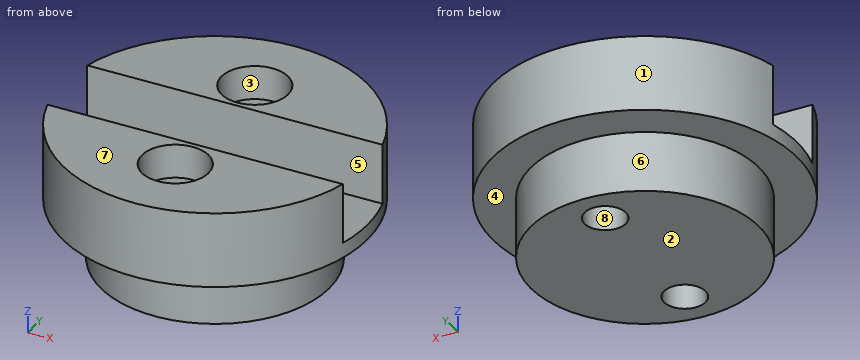
```python
from build123d import *

# Parameters (mm, degrees)
SKETCH1_R                                      = 9.525
BOSS_EXTRUDE1_DEPTH                            = 5.08
SKETCH2_R                                      = 12.7
BOSS_EXTRUDE2_DEPTH                            = 6.35
SKETCH3_W                                      = 25.4
SKETCH3_H                                      = 6.35
CUT_EXTRUDE1_DEPTH                             = 5.08
CBORE_FOR_4_SOCKET_HEAD_CAP_SCREW1_D           = 3.4544
CBORE_FOR_4_SOCKET_HEAD_CAP_SCREW1_CBORE_D     = 5.55752
CBORE_FOR_4_SOCKET_HEAD_CAP_SCREW1_CBORE_DEPTH = 2.8448


with BuildPart() as part:
    # Sketch1 → Boss-Extrude1 (new body)
    with BuildSketch(Plane.XY):
        Circle(SKETCH1_R)
    extrude(amount=BOSS_EXTRUDE1_DEPTH)

    # Sketch2 → Boss-Extrude2 (add)
    with BuildSketch(Plane.XY.offset(5.08)):
        Circle(SKETCH2_R)
    extrude(amount=BOSS_EXTRUDE2_DEPTH)

    # Sketch3 → Cut-Extrude1 (cut)
    with BuildSketch(Plane.XY.offset(11.43)):
        Rectangle(SKETCH3_W, SKETCH3_H)
    extrude(amount=-CUT_EXTRUDE1_DEPTH, mode=Mode.SUBTRACT)

    # CBORE for #4 Socket Head Cap Screw1 (through all)
    with Locations(Plane.XY.offset(11.43)):
        with Locations((0, -6.35), (0, 6.35)):
            CounterBoreHole(CBORE_FOR_4_SOCKET_HEAD_CAP_SCREW1_D / 2, CBORE_FOR_4_SOCKET_HEAD_CAP_SCREW1_CBORE_D / 2, CBORE_FOR_4_SOCKET_HEAD_CAP_SCREW1_CBORE_DEPTH)


solid = part.part
```
For this review, take the finished solid that the model builds, in its own axes (mm). Face numbers are marked on the shaded views. A direction names the side the tool comes from. Round coordinates to 2 decimals unless told otherwise and drop trailing zeros. Write each loop counter-clockwise with the first axis right and the second up, starting at its lowest first coordinate (ties: lowest second). Pieces come first, ordered by that corner, then holes. Notation, with made-up numbers: M -8,-36.5 L 17,-36.5 A18 cw 17,-12.5 Z; hole C 76.5,68 d4. An arc over 180 degrees is marked long. One line per item, written item: value. Start each with the question number.
(1) Wall thickness on line 1 (Y direction, x = 0, z = 10.65) (3 decimals); line 2 (Y direction, x = 0, z = 6); line 3 (Y direction, x = -0.25, z = 4.75): over which ranges is each line inside the solid? List them lowest first.
(2) We need section B-B (z = 9). Give the boundary of the cut face in (x, y) (3 decimals), and give its area (3 significant figures).
(3) We need section C-C (y = 0). Give the boundary of the cut face in (x, z) (3 decimals), and give its area (3 significant figures).
(4) The part is to be moulded in two halves that separate along X. For the marked faces 6, 7 and 8, say which applies: released by +X, released by -X, zero draft, split by the parting line, or undercut.
(5) Insertion check: pin 1 (1.7 mm diameter, centred on x = 0, y = 6, fed in from +Z); pin 2 (3 mm diameter, centred on y = -7.5, z = 9.5, fed in from +X); pin 3 (4 mm diameter, centred on y = -2, z = 2, fed in from -X) (3 decimals); pin 4 (4.5 mm diameter, centred on x = 0, y = -6.35, fed in from +Z). Each pin has a flat end and moves straight along its axis. Give the tip position at first contact, or say it passes through.
(6) We need section A-A (x = 0). Give the boundary of the cut face in (y, z) (3 decimals).
(7) Machinability: for the marked faces 1, 2, 3, 4 and 5, which of the approach directions +Z, -Z, +X, -X, +Y, -Y give a long, thin tool a straight path to every point of the face, cutting with its end or side? Answer none if there is none.
(8) We need section D-D (y = -6.35). Give the boundary of the cut face in (x, z), and give its area (3 significant figures).
Result:
1. line 1: -12.7 to -9.129, -3.571 to -3.175, 3.175 to 3.571, 9.129 to 12.7
1. line 2: -12.7 to -8.08, -4.62 to 4.62, 8.08 to 12.7
1. line 3: -9.52 to -8.06, -4.64 to 4.64, 8.06 to 9.52
2. outline: M -12.297,-3.175 A12.7 ccw 12.297,-3.175 Z; M -12.297,3.175 L 12.297,3.175 A12.7 ccw Z; hole C 0,-6.35 d5.558; hole C 0,6.35 d5.558
2. area: 299 mm²
3. outline: M -12.7,5.08 L -9.525,5.08 L -9.525,0 L 9.525,0 L 9.525,5.08 L 12.7,5.08 L 12.7,6.35 L -12.7,6.35 Z
3. area: 129 mm²
4. face 6: split by the parting line
4. face 7: zero draft
4. face 8: undercut
5. pin 1: through
5. pin 2: x = 11.19
5. pin 3: x = -9.525
5. pin 4: z = 8.59
6. outline: M -12.7,5.08 L -9.525,5.08 L -9.525,0 L -8.077,0 L -8.077,8.585 L -9.129,8.585 L -9.129,11.43 L -12.7,11.43 Z; M -4.623,0 L 4.623,0 L 4.623,8.585 L 3.571,8.585 L 3.571,11.43 L 3.175,11.43 L 3.175,6.35 L -3.175,6.35 L -3.175,11.43 L -3.571,11.43 L -3.571,8.585 L -4.623,8.585 Z; M 8.077,0 L 9.525,0 L 9.525,5.08 L 12.7,5.08 L 12.7,11.43 L 9.129,11.43 L 9.129,8.585 L 8.077,8.585 Z
7. face 1: +Z, -Z
7. face 2: -Z, +X, -X, +Y, -Y
7. face 3: +Z
7. face 4: -Z
7. face 5: +Z, +X, -X
8. outline: M -11,5.08 L -7.1,5.08 L -7.1,0 L -1.73,0 L -1.73,8.59 L -2.78,8.59 L -2.78,11.43 L -11,11.43 Z; M 1.73,0 L 7.1,0 L 7.1,5.08 L 11,5.08 L 11,11.43 L 2.78,11.43 L 2.78,8.59 L 1.73,8.59 Z
8. area: 166 mm²
